```python
from build123d import *

# Parameters (mm, degrees)
BOSS_EXTRUDE1_DEPTH = 6.35
SKETCH4_R           = 1.2
CUT_EXTRUDE3_DEPTH  = 2540
SKETCH129_R         = 0.775
CUT_EXTRUDE5_DEPTH  = 3
SKETCH130_R         = 0.775
CUT_EXTRUDE6_DEPTH  = 8
CUT_EXTRUDE7_START  = -8
SKETCH131_R         = 0.775
CUT_EXTRUDE7_DEPTH  = 8
CUT_EXTRUDE8_START  = -8
SKETCH132_R         = 0.775
CUT_EXTRUDE8_DEPTH  = 8
SKETCH133_R         = 1.6
CUT_EXTRUDE9_DEPTH  = 10
SKETCH134_R         = 1.6
CUT_EXTRUDE10_DEPTH = 10
SKETCH135_R         = 1.5
CUT_EXTRUDE11_DEPTH = 142.56384602
SKETCH136_W         = 21
SKETCH136_H         = 90
CUT_EXTRUDE12_DEPTH = 142.56384602


with BuildPart() as part:
    # Sketch1 → Boss-Extrude1 (new body)
    with BuildSketch(Plane(origin=(0, 0, 0), x_dir=(1, 0, 0), z_dir=(0, 1, 0))):
        Polygon((1, 83), (0, 83), (0, 17), (1, 17), (1, 1), (17, 1), (17, 0), (83, 0), (83, 1), (99, 1), (99, 17), (100, 17), (100, 83), (99, 83), (99, 99), (83, 99), (83, 100), (17, 100), (17, 99), (1, 99), align=None)
    extrude(amount=BOSS_EXTRUDE1_DEPTH)

    # Sketch4 → Cut-Extrude3 (cut, symmetric)
    with BuildSketch(Plane(origin=(-170.766523355, -217.05420542, -269.308617799), x_dir=(0, 0, -1), z_dir=(0, -1, 0))):
        with Locations((-179.303617798, 177.901523357)):
            Circle(SKETCH4_R)
        with Locations((-259.313617798, 177.901523357)):
            Circle(SKETCH4_R)
        with Locations((-256.773617797, 263.631523357)):
            Circle(SKETCH4_R)
        with Locations((-183.113617797, 263.631523357)):
            Circle(SKETCH4_R)
    extrude(amount=CUT_EXTRUDE3_DEPTH, both=True, mode=Mode.SUBTRACT)

    # Sketch129 → Cut-Extrude5 (cut)
    with BuildSketch(Plane(origin=(99, 0, 0), x_dir=(0, 0, -1), z_dir=(1, 0, 0))):
        with Locations((12.75, 3.175)):
            Circle(SKETCH129_R)
        with Locations((87.25, 3.175)):
            Circle(SKETCH129_R)
    extrude(amount=-CUT_EXTRUDE5_DEPTH, mode=Mode.SUBTRACT)

    # Sketch130 → Cut-Extrude6 (cut)
    with BuildSketch(Plane.XY.offset(-1)):
        with Locations((87.25, 3.175)):
            Circle(SKETCH130_R)
        with Locations((12.75, 3.175)):
            Circle(SKETCH130_R)
    extrude(amount=-CUT_EXTRUDE6_DEPTH, mode=Mode.SUBTRACT)

    # Sketch131 → Cut-Extrude7 (cut)
    with BuildSketch(Plane.ZY.offset(-1).offset(CUT_EXTRUDE7_START)):
        with Locations(Location((-12.75, 3.175, 0), (0, 0, 180))):
            Circle(SKETCH131_R)
        with Locations(Location((-87.25, 3.175, 0), (0, 0, 180))):
            Circle(SKETCH131_R)
    extrude(amount=CUT_EXTRUDE7_DEPTH, mode=Mode.SUBTRACT)

    # Sketch132 → Cut-Extrude8 (cut)
    with BuildSketch(Plane(origin=(0, 0, -99), x_dir=(-1, 0, 0), z_dir=(0, 0, -1)).offset(CUT_EXTRUDE8_START)):
        with Locations(Location((-87.25, 3.175, 0), (0, 0, 180))):
            Circle(SKETCH132_R)
        with Locations(Location((-12.75, 3.175, 0), (0, 0, 180))):
            Circle(SKETCH132_R)
    extrude(amount=CUT_EXTRUDE8_DEPTH, mode=Mode.SUBTRACT)

    # Sketch133 → Cut-Extrude9 (cut)
    with BuildSketch(Plane(origin=(0, 6.35, 0), x_dir=(1, 0, 0), z_dir=(0, 1, 0))):
        with Locations(Location((4.25, 95.75, 0), (0, 0, 270))):
            Circle(SKETCH133_R)
        with Locations(Location((4.25, 4.25, 0), (0, 0, 270))):
            Circle(SKETCH133_R)
        with Locations(Location((95.75, 95.75, 0), (0, 0, 270))):
            Circle(SKETCH133_R)
        with Locations(Location((95.75, 4.25, 0), (0, 0, 270))):
            Circle(SKETCH133_R)
    extrude(amount=-CUT_EXTRUDE9_DEPTH, mode=Mode.SUBTRACT)

    # Sketch134 → Cut-Extrude10 (cut)
    with BuildSketch(Plane(origin=(0, 6.35, 0), x_dir=(1, 0, 0), z_dir=(0, 1, 0))):
        with Locations(Location((92.865000001, 86.195000002, 0), (0, 0, 270))):
            Circle(SKETCH134_R)
        with Locations(Location((92.865000002, 12.535000002, 0), (0, 0, 270))):
            Circle(SKETCH134_R)
        with Locations(Location((7.135000002, 9.995000001, 0), (0, 0, 270))):
            Circle(SKETCH134_R)
        with Locations(Location((7.135000001, 90.005000001, 0), (0, 0, 270))):
            Circle(SKETCH134_R)
    extrude(amount=-CUT_EXTRUDE10_DEPTH, mode=Mode.SUBTRACT)

    # Sketch135 → Cut-Extrude11 (cut, through all)
    with BuildSketch(Plane.XZ):
        with Locations(Location((2.8068, -50, 0), (0, 0, 270))):
            Circle(SKETCH135_R)
        with Locations(Location((50, -2.8068, 0), (0, 0, 270))):
            Circle(SKETCH135_R)
        with Locations(Location((97.1932, -50, 0), (0, 0, 270))):
            Circle(SKETCH135_R)
        with Locations(Location((50, -97.1932, 0), (0, 0, 270))):
            Circle(SKETCH135_R)
    extrude(amount=-CUT_EXTRUDE11_DEPTH, mode=Mode.SUBTRACT)

    # Sketch136 → Cut-Extrude12 (cut, through all)
    with BuildSketch(Plane.XZ):
        with Locations((33.5, -50)):
            Rectangle(SKETCH136_W, SKETCH136_H)
    extrude(amount=-CUT_EXTRUDE12_DEPTH, mode=Mode.SUBTRACT)


solid = part.part
```
Model file for the job. Use its own axes, mm. A direction names the side the tool comes from. Give positions to 0.01 mm unless a question says otherwise; leave off trailing zeros. Order: outer loops, then holes, each group sorted by start corner. A loop starts at its lowest first (then second) coordinate and runs counter-clockwise, first axis right, second up.
1) 3-axis set-ups, long thin cutter, end or side, ignore diameter. For faces 4 (the flat face through (23, 3, -51)), 5 (the flat face through (9, 3, -99)), 6 (the flat face through (91, 3, -1)): which of +Z, -Z, +X, -X, +Y, -Y reach the whole face in a straight line?
2) Mould opens along X. For faces 1 (the cylindrical face through (4.32, 3.22, -97.35)), 2 (the flat face through (1, 3, -91)), 3 (the flat face through (49, 0, -51)) say: +X half, -X half, draft (parallel to the pull), parting line (faces both ways), or undercut.
3) Saw through at D-D, the plane y = 1. Count the separate pieces of the cut face and the enclosed holes in it, then the cut area to 3 significant figures.
4) Saw through at B-B, the plane x = 33. Write the cut outline in (y, z).
5) Wall check: probe 1 along Z at (x, y) = (93, 5); probe 2 along X at (y, z) = (1, -12.5); probe 3 along X at (y, z) = (3, -50). Give the ranges that are in metal, low to high.
6) Saw through at C-C, the plane x = 90. Write the cut outline in (y, z), then the cut area to 3 significant figures.
7) Pin check, flat tips, straight feed: pin 1 (0.5 mm diameter, centred on x = 99.5, y = 2.5, fed in from +Z); pin 2 (1.2 mm diameter, centred on y = 3.5, z = -87, fed in from -X); pin 3 (1 mm diameter, centred on x = 57.5, z = -11.5, fed in from -Y); pin 4 (1.2 mm diameter, centred on x = 13, y = 3, fed in from +Z). Stop position of each tip, or through.
8) Saw through at A-A, the plane z = -61.5. Write the cut outline in (x, y).
Computed:
1. face 4: +Y, -Y
1. face 5: -Z, -X, +Y, -Y
1. face 6: +Z, +X, +Y, -Y
2. face 1: undercut
2. face 2: -X half
2. face 3: draft
3. separate pieces: 1
3. enclosed holes: 13
3. area: 7,890 mm2
4. outline: (0, -100) - (6.35, -100) - (6.35, -95) - (0, -95) - close; (0, -5) - (6.35, -5) - (6.35, 0) - (0, 0) - close
5. probe 1: z = -99 to -87.79, -84.6 to -14.13, -10.94 to -1
5. probe 2: x = 1 to 23, 44 to 91.27, 94.46 to 99
5. probe 3: x = 0 to 1.31, 4.31 to 23, 44 to 95.69, 98.69 to 100
6. outline: (0, -99) - (6.35, -99) - (6.35, -1) - (0, -1) - close
6. area: 622 mm2
7. pin 1: stops at z = -17
7. pin 2: stops at x = 1
7. pin 3: stops at y = 0
7. pin 4: stops at z = -1
8. outline: (0, 0) - (23, 0) - (23, 6.35) - (0, 6.35) - close; (44, 0) - (100, 0) - (100, 6.35) - (44, 6.35) - close
